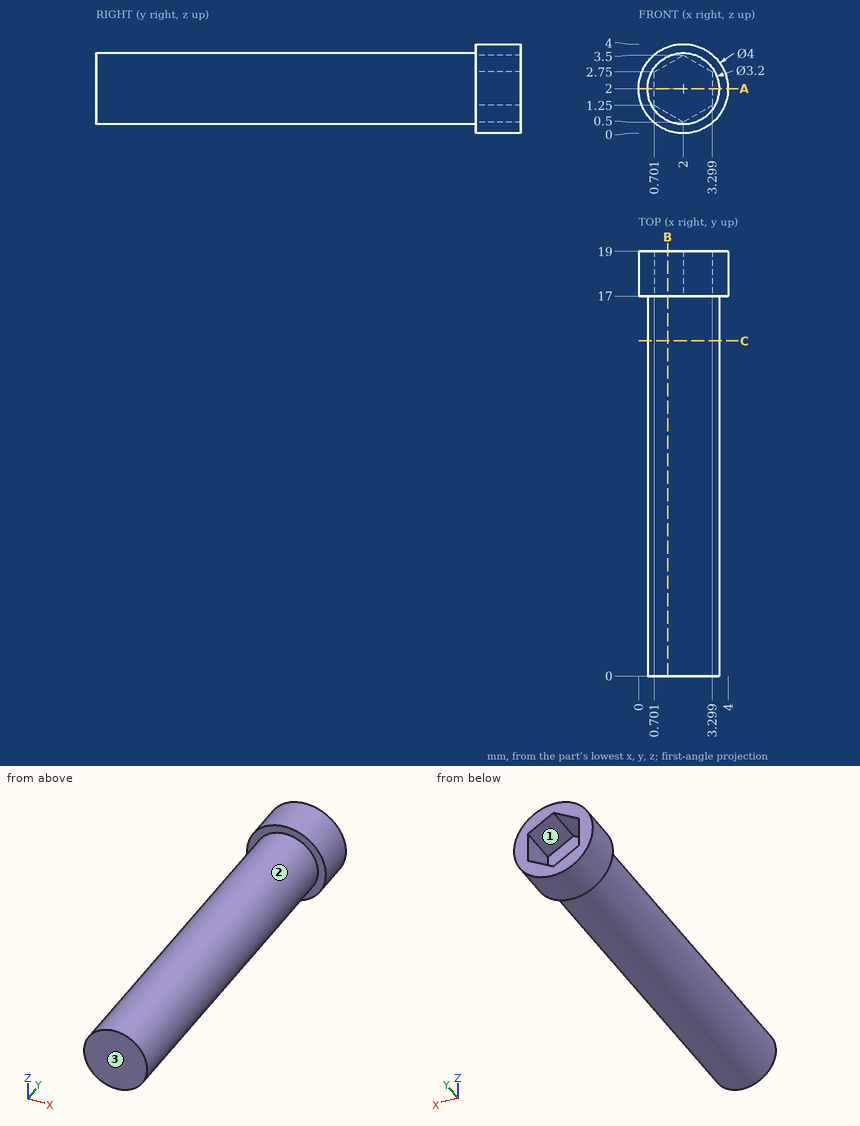
Here's the drawing with two shaded views (mm, measured from the low corner). I have some questions. Give positions to 0.01 mm unless a question says otherwise; leave off trailing zeros. Order: outer loops, then holes, each group sorted by start corner. A loop starts at its lowest first (then second) coordinate and runs counter-clockwise, first axis right, second up. Notation, with made-up numbers: (23, 37.5) - (76, 37.5) arc R38 cw to (76, 76.5) - close; hole circle Ø5 at (-10, 25.5). An arc over 180 degrees is marked (long way). Use a Markdown table: item, result. Add a question column.
Q1. Please list where these lines run through material, in increasing order: line 1 along Z through (x, y) = (1.45, 15.75); line 2 along Y through (x, z) = (3.75, 1.7); line 3 along X through (y, z) = (16.5, 1.9).
Q2. I'm going to push flat-ended pins straight in: pin 1 (1.5 mm diameter, centred on y = 3.5, z = 3, fed in from +X); pin 2 (2 mm diameter, centred on y = 6, z = 1.5, fed in from -X). Where does each tip first touch, or does it pass through?
Q3. If we section it at B-B on x = 1.3: Write out the boundary of the cut face in (y, z), plus the area to 3 significant figures.
Q4. If we mould it in two halves opening along Z, with no side actions, what happens to the marked faces 1, 2 and 3? For each: released by +Z, released by -Z, zero draft, split by the parting line, or undercut.
Q5. If we section it at C-C on y = 15: Write out the boundary of the cut face in (x, z).
Q6. If we section it at A-A on z = 2: Write out the boundary of the cut face in (x, y), plus the area to 3 significant figures.
Answers follow:
| question | item | result |
|---|---|---|
| 1 | line 1 | z = 0.5 to 3.5 |
| 1 | line 2 | y = 17 to 19 |
| 1 | line 3 | x = 0.4 to 3.6 |
| 2 | pin 1 | stops at x = 3.58 |
| 2 | pin 2 | stops at x = 0.4 |
| 3 | outline | (0, 0.56) - (17, 0.56) - (17, 0.13) - (19, 0.13) - (19, 0.9) - (17, 0.9) - (17, 3.1) - (19, 3.1) - (19, 3.87) - (17, 3.87) - (17, 3.44) - (0, 3.44) - close |
| 3 | area | 52.0 mm^2 |
| 4 | face 1 | undercut |
| 4 | face 2 | split by the parting line |
| 4 | face 3 | zero draft |
| 5 | outline | circle Ø3.2 at (2, 2) |
| 6 | outline | (0, 17) - (0.4, 17) - (0.4, 0) - (3.6, 0) - (3.6, 17) - (4, 17) - (4, 19) - (3.3, 19) - (3.3, 17) - (0.7, 17) - (0.7, 19) - (0, 19) - close |
| 6 | area | 57.2 mm^2 |
